Work out the finished part from the listing and answer in its coordinate system (mm). Face numbers are marked on the shaded views. Coordinates: 2 decimals unless noted, no trailing zeros. Loops run counter-clockwise (first coordinate to the right, second up) from the corner with the lowest first, then second, coordinate; pieces in that order, holes last. Notation, with made-up numbers: (-4.5, 86) - (30.5, 86) arc R12 cw to (30.5, 97) - close; hole circle Ø3 at (35.25, 64.25). An arc over 180 degrees is marked (long way). Write each question's results on one line, items separated by ' | '. Start each with the question number.
1. Determine the mould class of the marked faces 1 and 2 for opening direction Z: released by +Z, released by -Z, zero draft, split by the parting line, or undercut.
2. A cutting plane is placed at D-D on z = -1.7. Determine the outline of the cut face in (x, y).
3. A cutting plane is placed at A-A on z = -2.55. Determine the outline of the cut face in (x, y), then the cut area to 3 significant figures.
4. Each of these flat-tipped pins is pushed along its axis until it touches: P1, Ø6, axis at x = 1, y = 4, coming from the -Z side; P2, Ø0.6, axis at y = -6.5, z = -0.5, coming from the +X side; P3, Ø1.1, axis at x = 5.5, z = -1.5, coming from the -Y side. Where does it stop, or does it pass through?
5. A cutting plane is placed at C-C on y = -6.7. Determine the outline of the cut face in (x, z), then the cut area to 3 significant figures.
6. A cutting plane is placed at B-B on x = 1.75. Determine the outline of the cut face in (y, z), then the cut area to 3 significant figures.
7. Find the intervals of material crossed by line 1 along Y through (x, z) = (-5.25, -0.9); line 2 along X through (y, z) = (-8, -3); line 3 along Z through (x, y) = (5.5, 8.25), in increasing order. Write a range as [from, to].
from build123d import *

# Parameters (mm, degrees)
SKETCH006_W     = 12
SKETCH006_H     = 18.65
PAD002_DEPTH    = 2.25
SKETCH007_W     = 7.6
SKETCH007_H     = 3.7
PAD003_DEPTH    = 1.1
SKETCH008_W     = 0.5
SKETCH008_H     = 1.8
PAD004_DEPTH    = 1.35
POCKET003_DEPTH = 1


with BuildPart() as part:
    # Sketch006 → Pad002 (new body, symmetric)
    with BuildSketch(Plane.XY):
        with Locations((0, -0.325)):
            Rectangle(SKETCH006_W, SKETCH006_H)
    extrude(amount=PAD002_DEPTH, both=True)

    # Sketch007 (on Face3 of Pad002) → Pad003 (join)
    with BuildSketch(Plane.XZ.offset(9.65)):
        with Locations((0, -1.85)):
            Rectangle(SKETCH007_W, SKETCH007_H)
    extrude(amount=PAD003_DEPTH)

    # Sketch008 (on Face4 of Pad003) → Pad004 (join)
    with BuildSketch(Plane(origin=(0, 0, -2.25), x_dir=(1, 0, 0), z_dir=(0, 0, -1))):
        with Locations((-5.7, 8.65)):
            Rectangle(SKETCH008_W, SKETCH008_H)
    pad004 = extrude(amount=PAD004_DEPTH)

    # Mirrored: Pad004 across Sketch008 V_Axis
    add(pad004.mirror(Plane(origin=(0, 0, -2.25), x_dir=(0, 0, -1), z_dir=(1, 0, 0))))

    # Sketch009 (on Face3 of Mirrored) → Pocket003 (cut)
    with BuildSketch(Plane.YZ.offset(6)):
        with BuildLine():
            ThreePointArc((-5.75, -0.95), (-6.7, 0), (-7.65, -0.95))
            Line((-7.65, -2.95), (-7.65, -0.95))
            Line((-5.75, -2.95), (-7.65, -2.95))
            Line((-5.75, -0.95), (-5.75, -2.95))
        make_face()
    pocket003 = extrude(amount=-POCKET003_DEPTH, mode=Mode.SUBTRACT)

    # Mirrored001: Pocket003 across YZ
    add(pocket003.mirror(Plane.YZ), mode=Mode.SUBTRACT)


solid = part.part
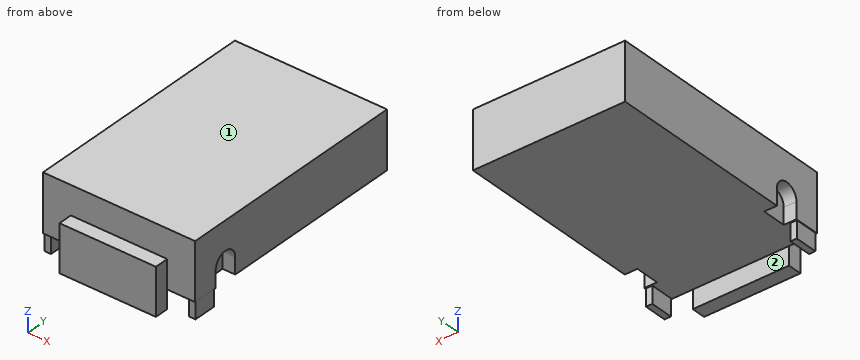
Values:
1) face 1: released by +Z | face 2: zero draft
2) outline: (-6, -9.65) - (-3.8, -9.65) - (-3.8, -10.75) - (3.8, -10.75) - (3.8, -9.65) - (6, -9.65) - (6, -7.65) - (5, -7.65) - (5, -5.75) - (6, -5.75) - (6, 9) - (-6, 9) - (-6, -5.75) - (-5, -5.75) - (-5, -7.65) - (-6, -7.65) - close
3) outline: (-5.95, -9.55) - (-5.45, -9.55) - (-5.45, -7.75) - (-5.95, -7.75) - close; (-3.8, -10.75) - (3.8, -10.75) - (3.8, -9.65) - (-3.8, -9.65) - close; (5.45, -9.55) - (5.95, -9.55) - (5.95, -7.75) - (5.45, -7.75) - close | area: 10.2 mm^2
4) P1: z = -2.25 | P2: x = 5 | P3: y = -9.65
5) outline: (-6, 0) - (-5, 0) - (-5, -2.25) - (5, -2.25) - (5, 0) - (6, 0) - (6, 2.25) - (-6, 2.25) - close | area: 49.5 mm^2
6) outline: (-10.75, -3.7) - (-9.65, -3.7) - (-9.65, -2.25) - (9, -2.25) - (9, 2.25) - (-9.65, 2.25) - (-9.65, 0) - (-10.75, 0) - close | area: 88.0 mm^2
7) line 1: [-9.65, -7.65], [-5.75, 9] | line 2: [-5.95, -5.45], [5.45, 5.95] | line 3: [-2.25, 2.25]
